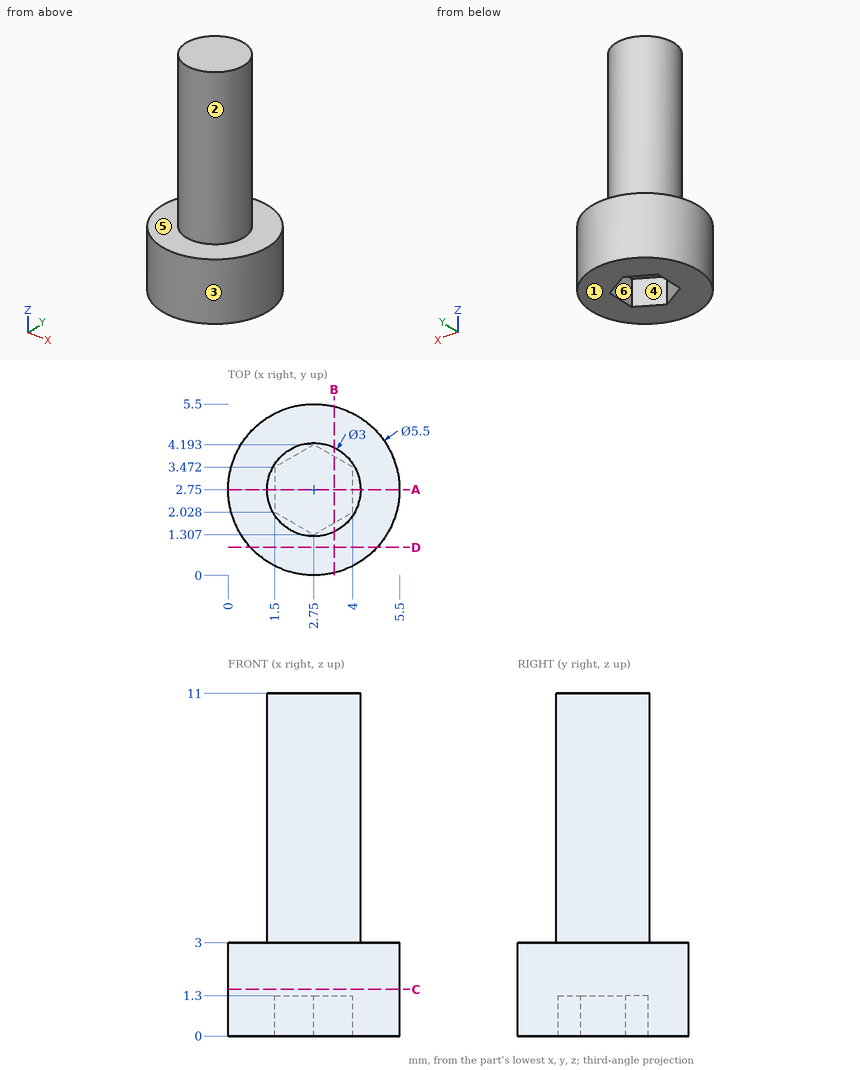
Job drawing, mm, ordinate dimensions from the low corner. One solid piece. A direction names the side the tool comes from. Give positions to 0.01 mm unless a question says otherwise; leave off trailing zeros. Order: outer loops, then holes, each group sorted by start corner. A loop starts at its lowest first (then second) coordinate and runs counter-clockwise, first axis right, second up. Notation, with made-up numbers: M 9,44 L 60,44 A25 ccw 60,63 Z; hole C -24,60 d3. An arc over 180 degrees is marked long. Return JSON: item names as keys, results as strings.
Q1. Band-saw the part on C-C (z = 1.5). Give the cut face in (x, y).
Answer list:
{"outline": "C 2.75,2.75 d5.5"}
Q2. Two-plate mould, pull along Y, no slides. Class the marked faces 3, 4, 5 and 6: pulls with the +Y half, pulls with the -Y half, needs draft (parallel to the pull), parting line crosses it, or undercut.
Answer list:
{"face 3": "parting line crosses it", "face 4": "undercut", "face 5": "needs draft", "face 6": "undercut"}
Q3. Wall check: probe 1 along Z at (x, y) = (0.9, 2.55); probe 2 along X at (y, z) = (2.05, 1); probe 3 along Z at (x, y) = (3.4, 1.75). Give the ranges that are in metal, low to high. Write a range as from..to.
Answer list:
{"probe 1": "z = 0..3", "probe 2": "x = 0.09..1.5, 4..5.41", "probe 3": "z = 1.3..11"}
Q4. Flat gauge pins, fed straight in: pin 1 (1.5 mm diameter, centred on x = 2.5, z = 5.5, fed in from +Y); pin 2 (2 mm diameter, centred on x = 4.5, z = 8, fed in from +Y); pin 3 (0.8 mm diameter, centred on x = 3, y = 3, fed in from -Z). Where does each tip first touch, or does it go through?
Answer list:
{"pin 1": "stops at y = 4.25", "pin 2": "stops at y = 4.05", "pin 3": "stops at z = 1.3"}
Q5. Band-saw the part on A-A (y = 2.75). Give the cut face in (x, z).
Answer list:
{"outline": "M 0,0 L 1.5,0 L 1.5,1.3 L 4,1.3 L 4,0 L 5.5,0 L 5.5,3 L 4.25,3 L 4.25,11 L 1.25,11 L 1.25,3 L 0,3 Z"}
Q6. Band-saw the part on B-B (x = 3.4). Give the cut face in (y, z), then the cut area to 3 significant figures.
Answer list:
{"outline": "M 0.08,0 L 1.68,0 L 1.68,1.3 L 3.82,1.3 L 3.82,0 L 5.42,0 L 5.42,3 L 4.1,3 L 4.1,11 L 1.4,11 L 1.4,3 L 0.08,3 Z", "area": "34.9 mm^2"}
Q7. Band-saw the part on D-D (y = 0.9). Give the cut face in (x, z) (1 decimal).
Answer list:
{"outline": "M 0.7,0 L 4.8,0 L 4.8,3 L 0.7,3 Z"}
Q8. 3-axis set-ups, long thin cutter, end or side, ignore diameter. For the marked faces 1 and 2: which of +Z, -Z, +X, -X, +Y, -Y reach the whole face in a straight line?
Answer list:
{"face 1": "-Z, +X, -X, +Y, -Y", "face 2": "+Z"}
